from build123d import *

# Parameters (mm, degrees)
SUSP_FR_LCA_FRONT_LEG_PROFILE_R  = 9.525
SUSP_FR_LCA_REAR_LEG_START       = 194.971257269
SUSP_FR_LCA_REAR_LEG_OUTLINE_R   = 9.525
SUSP_FR_LCA_REAR_LEG_DEPTH       = 392.368202981
SUSP_FR_LCA_REAR_LEG_START_2     = 587.33946025
SUSP_FR_LCA_REAR_LEG_2_OUTLINE_R = 9.525
SUSP_FR_LCA_REAR_LEG_2_DEPTH     = 13.53250199
SUSP_FR_LCA_REAR_LEG_START_3     = 523.39106775
SUSP_FR_LCA_REAR_LEG_3_OUTLINE_W = 26
SUSP_FR_LCA_REAR_LEG_3_OUTLINE_H = 23
SUSP_FR_LCA_REAR_LEG_3_DEPTH     = 11.60893225
SUSP_FR_LCA_BUSH_FRONT_PROFILE_R = 14
SUSP_FR_LCA_BUSH_REAR_PROFILE_R  = 14


with BuildPart() as part:
    # SUSP_FR_LCA_front_leg: sweep along a curve in space
    with BuildLine() as susp_fr_lca_front_leg_path:
        Line((205, -240.84, -42.383), (582, -130.461196, -55))
    # SUSP_FR_LCA_front_leg profile (on start of the path) → SUSP_FR_LCA_front_leg (sweep)
    with BuildSketch(Plane(origin=(205, -240.84, -42.383), x_dir=(-0.2809863080066093, 0.9597117768959672, 0), z_dir=(0.9592171404331008, 0.28084148736685866, -0.03210196992266429))):
        Circle(SUSP_FR_LCA_FRONT_LEG_PROFILE_R)
    sweep(path=susp_fr_lca_front_leg_path.line)

    # SUSP_FR_LCA_rear_leg: read off the stored shape, not the designer's step
    # SUSP_FR_LCA_rear_leg outline → SUSP_FR_LCA_rear_leg (add)
    with BuildSketch(Plane(origin=(0, 0, 0), x_dir=(0.3266773785489796, 0.9450726759891053, -0.01093286070332221), z_dir=(0.9445438654680327, -0.3268602715210149, -0.031610901725756396)).offset(SUSP_FR_LCA_REAR_LEG_START)):
        with Locations((67.432230038, -35.502420765)):
            Circle(SUSP_FR_LCA_REAR_LEG_OUTLINE_R)
    extrude(amount=SUSP_FR_LCA_REAR_LEG_DEPTH)

    # SUSP_FR_LCA_rear_leg 2 outline → SUSP_FR_LCA_rear_leg 2 (add)
    with BuildSketch(Plane(origin=(0, 0, 0), x_dir=(0.3266773785489796, 0.9450726759891053, -0.01093286070332221), z_dir=(0.9445438654680327, -0.3268602715210149, -0.031610901725756396)).offset(SUSP_FR_LCA_REAR_LEG_START_2)):
        with Locations((67.432230038, -35.502420765)):
            Circle(SUSP_FR_LCA_REAR_LEG_2_OUTLINE_R)
    extrude(amount=SUSP_FR_LCA_REAR_LEG_2_DEPTH)

    # SUSP_FR_LCA_rear_leg 3 outline → SUSP_FR_LCA_rear_leg 3 (cut)
    with BuildSketch(Plane(origin=(0, 0, 0), x_dir=(-0.28068434396715386, 0.959754165905817, 0.009393619012821172), z_dir=(0.9592171404331008, 0.2808414873668589, -0.03210196992266429)).offset(SUSP_FR_LCA_REAR_LEG_START_3)):
        with Locations((-289, -35.5)):
            Rectangle(SUSP_FR_LCA_REAR_LEG_3_OUTLINE_W, SUSP_FR_LCA_REAR_LEG_3_OUTLINE_H)
    extrude(amount=SUSP_FR_LCA_REAR_LEG_3_DEPTH, mode=Mode.SUBTRACT)

    # SUSP_FR_LCA_bush_front: sweep along a curve in space
    with BuildLine() as susp_fr_lca_bush_front_path:
        Line((205, -255.84, -42.383), (205, -225.84, -42.383))
    # SUSP_FR_LCA_bush_front profile (on start of the path) → SUSP_FR_LCA_bush_front (sweep)
    with BuildSketch(Plane(origin=(205, -255.84, -42.383), x_dir=(0, 0, 1), z_dir=(0, 1, 0))):
        Circle(SUSP_FR_LCA_BUSH_FRONT_PROFILE_R)
    sweep(path=susp_fr_lca_bush_front_path.line)

    # SUSP_FR_LCA_bush_rear: sweep along a curve in space
    with BuildLine() as susp_fr_lca_bush_rear_path:
        Line((205, -15, -42.383), (205, 15, -42.383))
    # SUSP_FR_LCA_bush_rear profile (on start of the path) → SUSP_FR_LCA_bush_rear (sweep)
    with BuildSketch(Plane(origin=(205, -15, -42.383), x_dir=(0, 0, 1), z_dir=(0, 1, 0))):
        Circle(SUSP_FR_LCA_BUSH_REAR_PROFILE_R)
    sweep(path=susp_fr_lca_bush_rear_path.line)


solid = part.part
Verification items for the finished model (mm, model axes). A direction names the side the tool comes from. Coordinates: 2 decimals unless noted, no trailing zeros. Write each loop counter-clockwise with the first axis right and the second up, starting at its lowest first coordinate (ties: lowest second). Pieces come first, ordered by that corner, then holes. Notation, with made-up numbers: (56, 27) - (111, 27) arc R26 ccw to (111, 63) - close; hole circle Ø1 at (-12, -19.75). An arc over 180 degrees is marked (long way). Answer as a JSON object with one key per item and string values.
(1) Cross-section at A-A on x = 205. Record the cut outline in (y, z).
Report:
{"outline": "(-255.84, -56.38) - (-225.84, -56.38) - (-225.84, -28.38) - (-255.84, -28.38) - close; (-15, -56.38) - (15, -56.38) - (15, -28.38) - (-15, -28.38) - close"}
(2) Thickness scan on line 1 along Y through (x, z) = (278.5, -46); line 2 along Y through (x, z) = (343, -41); line 3 along Z through (x, y) = (460, -97.5). Record the ranges inside material, lowest first.
Report:
{"line 1": "-229.16 to -209.46, -35.45 to -15.44", "line 2": "-208.2 to -192.79, -55.51 to -39.86", "line 3": "-54.78 to -47.24"}
(3) Tool access check on faces 3 (the flat face through (205, -15, -43)), 4 (the flat face through (205, 15, -43)). Record the directions out of +Z, -Z, +X, -X, +Y, -Y that give a thin tool (end or side, any length) a straight path to the whole face; none if there is none.
Report:
{"face 3": "+Z, -Z, -X", "face 4": "+Z, -Z, +X, -X, +Y"}
(4) Gauge pin test, flat ends, axial feed: pin 1 Ø10 at (x, y) = (424.5, -167.5) entering from -Z; pin 2 Ø8 at (x, z) = (292.5, -55) entering from +Y; pin 3 Ø5 at (x, z) = (533, -44) entering from -Y. Record the tip position at first contact, or that the pin passes through.
Report:
{"pin 1": "z = -58.59", "pin 2": "y = -22.02", "pin 3": "y = -151.89"}
(5) Mould release check, pull along X, two halves, no side actions. Record for faces 1 (the flat face through (205, -225.84, -43)), 2 (the cylindrical face through (582.308, -140.645, -54.94)): pulls with the +X half, pulls with the -X half, needs draft (parallel to the pull), parting line crosses it, or undercut.
Report:
{"face 1": "needs draft", "face 2": "undercut"}
